Can you work these out from the model? Positions are in its coordinate system, mm. A direction names the side the tool comes from. Round coordinates to 2 decimals unless told otherwise and drop trailing zeros. Order: outer loops, then holes, each group sorted by start corner. A loop starts at its lowest first (then second) coordinate and runs counter-clockwise, first axis right, second up.
Q1. If we section it at A-A (y = 58.5): Please give me the cut outline in (x, z).
Q2. Will these pins go through, and if not, where does the flat tip stop? P1, Ø10, axis at x = 39, y = 47, coming from the -Z side; P2, Ø8, axis at x = 39.5, y = 60.5, coming from the -Z side.
Q3. If we section it at C-C (y = 8): Please give me the cut outline in (x, z), plus the area to 3 significant figures.
Q4. If I drill on line 1 (Y direction, x = 35, z = 0.55); line 2 (Y direction, x = 45.25, z = 2.15); line 3 (Y direction, x = 45, z = 0.6), over which ranges is the centre line in solid material (lowest first)?
Q5. If we section it at B-B (x = 12): Please give me the cut outline in (y, z).
Q6. For faces 1 (the face through (34, 31, 3)), 2 (the face through (45, 53, 1)), which set-ups out of +Z, -Z, +X, -X, +Y, -Y let a thin tool reach every point of the face, with its end or its side?
from build123d import *

# Parameters (mm, degrees)
SKETCH_1_W          = 70
SKETCH_1_H          = 80
EXTRUDE_1_DEPTH     = 3
CUT_EXTRUDE_1_REACH = 108.344
SKETCH_2_R          = 0.6
SKETCH_2_R_2        = 11
SKETCH_3_R          = 12
CUT_EXTRUDE_2_DEPTH = 2
EXTRUDE_2_DEPTH     = 3


with BuildPart() as part:
    # 草图1 → 凸台-拉伸1 (new body)
    with BuildSketch(Plane.XY):
        with Locations((35, 40)):
            Rectangle(SKETCH_1_W, SKETCH_1_H)
    extrude(amount=EXTRUDE_1_DEPTH)

    # 草图2 → 切除-拉伸1 (cut, up to next)
    with BuildSketch(Plane.XY.offset(3), mode=Mode.PRIVATE) as cut_extrude_1_sk1:
        with Locations((24.75, 50)):
            Circle(SKETCH_2_R)
    cut_extrude_1_tool1 = extrude(cut_extrude_1_sk1.sketch, amount=-CUT_EXTRUDE_1_REACH, mode=Mode.PRIVATE) & part.part
    # 草图2 → 切除-拉伸1 (cut, up to next)
    with BuildSketch(Plane.XY.offset(3), mode=Mode.PRIVATE) as cut_extrude_1_sk2:
        with Locations((45.25, 50)):
            Circle(SKETCH_2_R)
    cut_extrude_1_tool2 = extrude(cut_extrude_1_sk2.sketch, amount=-CUT_EXTRUDE_1_REACH, mode=Mode.PRIVATE) & part.part
    # 草图2 → 切除-拉伸1 (cut, up to next)
    with BuildSketch(Plane.XY.offset(3), mode=Mode.PRIVATE) as cut_extrude_1_sk3:
        with Locations((45.25, 29.3)):
            Circle(SKETCH_2_R)
    cut_extrude_1_tool3 = extrude(cut_extrude_1_sk3.sketch, amount=-CUT_EXTRUDE_1_REACH, mode=Mode.PRIVATE) & part.part
    # 草图2 → 切除-拉伸1 (cut, up to next)
    with BuildSketch(Plane.XY.offset(3), mode=Mode.PRIVATE) as cut_extrude_1_sk4:
        with Locations((24.75, 29.3)):
            Circle(SKETCH_2_R)
    cut_extrude_1_tool4 = extrude(cut_extrude_1_sk4.sketch, amount=-CUT_EXTRUDE_1_REACH, mode=Mode.PRIVATE) & part.part
    # 草图2 → 切除-拉伸1 (cut, up to next)
    with BuildSketch(Plane.XY.offset(3), mode=Mode.PRIVATE) as cut_extrude_1_sk5:
        with Locations((35, 58.5)):
            Circle(SKETCH_2_R_2)
    cut_extrude_1_tool5 = extrude(cut_extrude_1_sk5.sketch, amount=-CUT_EXTRUDE_1_REACH, mode=Mode.PRIVATE) & part.part
    add(cut_extrude_1_tool1.solids().sort_by_distance((24.75, 50, 3))[0], mode=Mode.SUBTRACT)
    add(cut_extrude_1_tool2.solids().sort_by_distance((45.25, 50, 3))[0], mode=Mode.SUBTRACT)
    add(cut_extrude_1_tool3.solids().sort_by_distance((45.25, 29.3, 3))[0], mode=Mode.SUBTRACT)
    add(cut_extrude_1_tool4.solids().sort_by_distance((24.75, 29.3, 3))[0], mode=Mode.SUBTRACT)
    add(cut_extrude_1_tool5.solids().sort_by_distance((35, 58.5, 3))[0], mode=Mode.SUBTRACT)

    # 草图3 → 切除-拉伸2 (cut)
    with BuildSketch(Plane.XY.offset(3)):
        with Locations((35, 58.5)):
            Circle(SKETCH_3_R)
    extrude(amount=-CUT_EXTRUDE_2_DEPTH, mode=Mode.SUBTRACT)

    # 草图5 → 凸台-拉伸2 (add)
    with BuildSketch(Plane(origin=(0, 0, 0), x_dir=(-1, 0, 0), z_dir=(0, 0, -1))):
        Polygon((-75, 80), (-70, 80), (-70, 0), align=None)
        Polygon((0, 0), (5, 80), (0, 80), align=None)
        with BuildLine():
            Line((0, 0), (-35, 0))
            Line((-35, 0), (-35, -20.311288741))
            ThreePointArc((-35, -20.311288741), (-14.766683105, -14.865640499), (0, 0))
        make_face()
        with BuildLine():
            Line((-35, -20.311288741), (-35, 0))
            Line((-35, 0), (-70, 0))
            ThreePointArc((-70, 0), (-55.233316895, -14.865640499), (-35, -20.311288741))
        make_face()
        with BuildLine():
            Line((0, 0), (-35, 0))
            Line((-35, 0), (-35, -20.311288741))
            ThreePointArc((-35, -20.311288741), (-14.766683105, -14.865640499), (0, 0))
        make_face()
        with BuildLine():
            Line((-35, -20.311288741), (-35, 0))
            Line((-35, 0), (-70, 0))
            ThreePointArc((-70, 0), (-55.233316895, -14.865640499), (-35, -20.311288741))
        make_face()
    extrude(amount=-EXTRUDE_2_DEPTH)


solid = part.part
Solution:
1. outline: (-3.66, 0) - (24, 0) - (24, 1) - (23, 1) - (23, 3) - (-3.66, 3) - close; (46, 0) - (73.66, 0) - (73.66, 3) - (47, 3) - (47, 1) - (46, 1) - close
2. P1: stops at z = 0
2. P2: passes through
3. outline: (-0.5, 0) - (70.5, 0) - (70.5, 3) - (-0.5, 3) - close
3. area: 213 mm2
4. line 1: y = -20.31 to 47.5, 69.5 to 80
4. line 2: y = -18.99 to 28.7, 29.9 to 49.4, 50.6 to 52.26, 64.74 to 80
4. line 3: y = -19.05 to 28.75, 29.85 to 49.45, 50.55 to 53.92, 63.08 to 80
5. outline: (-13.11, 0) - (80, 0) - (80, 3) - (-13.11, 3) - close
6. face 1: +Z, +X, -X, +Y, -Y
6. face 2: +Z
